```python
from build123d import *

# Parameters (mm, degrees)
F0_W     = 254
F0_H     = 152.4
F1_DEPTH = 127
F2_R     = 25.4
F6_R     = 14.6864926798
F6_R_2   = 7.661429367
F6_R_3   = 15.1712278357
F6_R_4   = 10.7604265213
F7_DEPTH = 101.6


with BuildPart() as f1:
    # F0 (on Right) → F1 (new body)
    with BuildSketch(Plane.YZ):
        with Locations((127, 76.2)):
            Rectangle(F0_W, F0_H)
    extrude(amount=F1_DEPTH)

    # F2
    f2_edges = [f1.edges().sort_by_distance(p)[0] for p in [
        (63.5, 254, 152.4),
        (63.5, 0, 152.4),
        (0, 127, 152.4),
        (127, 127, 152.4),
        (63.5, 254, 0),
        (0, 254, 76.2),
        (127, 254, 76.2),
        (127, 0, 76.2),
        (127, 127, 0),
        (0, 0, 76.2),
        (0, 127, 0),
        (63.5, 0, 0),
    ]]
    fillet(f2_edges, radius=F2_R)

    # F4 (on offset) → F5 (revolve, cut)
    with BuildSketch(Plane.XY.offset(127)):
        with BuildLine():
            Line((63.5, 158.75), (63.5, 234.95))
            ThreePointArc((63.5, 234.95), (25.4, 196.85), (63.5, 158.75))
        make_face()
    revolve(axis=Axis((63.5, 196.85, 127), (0, -1, 0)), mode=Mode.SUBTRACT)

    # F6 (on face) → F7 (join)
    with BuildSketch(Plane(origin=(0, 0, 0), x_dir=(1, 0, 0), z_dir=(0, 0, -1))):
        with Locations((47.7847903967, -54.721660912)):
            Circle(F6_R)
        with Locations((89.0330970287, -54.2733110487)):
            Circle(F6_R_2)
        with Locations((45.5430299044, -199.9874413013)):
            Circle(F6_R_3)
        with Locations((82.7561765909, -198.1940418482)):
            Circle(F6_R_4)
    extrude(amount=F7_DEPTH)


solid = f1.part
```
Here's how the part is built. I have some questions about the finished solid (model axes, mm). A direction names the side the tool comes from. Give positions to 0.01 mm unless a question says otherwise; leave off trailing zeros. Loops run counter-clockwise (first coordinate to the right, second up) from the corner with the lowest first, then second, coordinate; pieces in that order, holes last. Notation, with made-up numbers: (34.25, -4.5) -> (90.25, -4.5) arc R23 cw to (90.25, 30.5) -> close; hole circle Ø2 at (-32.75, 7.5). An arc over 180 degrees is marked (long way). Use one line per item in the form item = value. Start each with the question number.
1) Please list where these lines run through material, in increasing order: line 1 along Z through (x, y) = (86, 136); line 2 along Y through (x, z) = (49.5, 145.5); line 3 along Y through (x, z) = (32, 137).
2) Imagine slicing it at D-D (z = -13). Please give me the cut outline in (x, y), then the cut area to 3 significant figures.
3) For P1, Ø10, axis at x = 103.5, z = -38.5, coming from the -Y side; P2, Ø4, axis at x = 109.5, z = 133, coming from the +Y side; P3, Ø6, axis at x = 91.5, y = 162, coming from the +Z side; P4, Ø5, axis at y = 205.5, z = 0.5, coming from the -X side (3 decimals), each with a flat end and sliding along its axis, tell me the tip position at first contact or that it passes through.
4) Imagine slicing it at C-C (x = 40.5). Please give me the cut outline in (y, z), then the cut area to 3 significant figures.
5) Which directions (+Z, -Z, +X, -X, +Y, -Y) give clear straight access to the entire face, cutting with the end or side of a thin tool? Please do faces 5 (the face through (63, 254, 75)), 6 (the face through (81.38, 53.94, -50.09)).
6) Imagine slicing it at B-B (z = 96.5). Please give me the cut outline in (x, y), then the cut area to 3 significant figures.
7) Thinking about a two-plate mould opening in X: for faces 1 (the face through (7.64, 128.42, 7.24)), 2 (the face through (127, 126, 77)), 3 (the face through (64.03, 246.76, 144.76)), 4 (the face through (80.424, 208.699, -50.089)), which applies, +X half, -X half, draft (parallel to the pull), parting line (faces both ways), or undercut?
8) Imagine slicing it at A-A (y = 144.5). Please give me the cut outline in (x, z), then the cut area to 3 significant figures.
Check values:
q1.line_1 = 0 to 152.4
q1.line_2 = 8 to 166.63, 227.07 to 246
q1.line_3 = 2.05 to 177.89, 215.81 to 251.95
q2.outline = circle Ø30.34 at (45.54, 199.99); circle Ø29.37 at (47.78, 54.72); circle Ø21.52 at (82.76, 198.19); circle Ø15.32 at (89.03, 54.27)
q2.area = 1,950 mm^2
q3.P1 = through
q3.P2 = 252.73
q3.P3 = 152.4
q3.P4 = 13.425
q4.outline = (0, 25.4) arc R25.4 ccw to (25.4, 0) -> (41.97, 0) -> (41.97, -101.6) -> (67.47, -101.6) -> (67.47, 0) -> (185.68, 0) -> (185.68, -101.6) -> (214.3, -101.6) -> (214.3, 0) -> (228.6, 0) arc R25.4 ccw to (254, 25.4) -> (254, 127) arc R25.4 ccw to (228.6, 152.4) -> (213.51, 152.4) arc R30.37 cw (long way) to (180.19, 152.4) -> (25.4, 152.4) arc R25.4 ccw to (0, 127) -> close
q4.area = 40,900 mm^2
q5.face_5 = +Z, -Z, +X, -X, +Y
q5.face_6 = -Z
q6.outline = (0, 25.4) arc R25.4 ccw to (25.4, 0) -> (101.6, 0) arc R25.4 ccw to (127, 25.4) -> (127, 228.6) arc R25.4 ccw to (101.6, 254) -> (25.4, 254) arc R25.4 ccw to (0, 228.6) -> close; hole circle Ø45.67 at (63.5, 196.85)
q6.area = 30,100 mm^2
q7.face_1 = -X half
q7.face_2 = +X half
q7.face_3 = draft
q7.face_4 = undercut
q8.outline = (0, 25.4) arc R25.4 ccw to (25.4, 0) -> (101.6, 0) arc R25.4 ccw to (127, 25.4) -> (127, 127) arc R25.4 ccw to (101.6, 152.4) -> (25.4, 152.4) arc R25.4 ccw to (0, 127) -> close
q8.area = 18,800 mm^2
